Solid Edge part; units mm, degrees
sketch "Sketch1" plane through (0, 0, 0) normal (0, 0, 1) x (1, 0, 0)
  line L0 (-3.8849, 0.05) -> (2.2199, 4.5741)
  line L1 (2.2199, 4.5741) -> (2.2199, -4.4741)
  line L2 (-3.8849, 0.05) -> (2.2199, -4.4741)
extrude "Protrusion1" add sketch "Sketch1" along normal blind 0.1
sketch "Sketch2" plane through (-0.8325, 0.05, 0.1) normal (0, 0, 1) x (0, 1, 0)
  line L0 (-0.79, -3.0024) -> (0.76, -3.0024)
  line L1 (0.76, -3.0024) -> (0.76, -1.0024)
  line L2 (0.76, -1.0024) -> (-0.79, -1.0024)
  line L3 (-0.79, -1.0024) -> (-0.79, -3.0024)
  dimension "D1" = 0.76
  dimension "D2" = 0.79
extrude "Cutout1" cut sketch "Sketch2" against normal through all
Geometry check sheet. Reference: the model listing, model coordinates, mm. Give positions to 0.01 mm unless a question says otherwise; leave off trailing zeros. Order: outer loops, then holes, each group sorted by start corner. A loop starts at its lowest first (then second) coordinate and runs counter-clockwise, first axis right, second up. Notation, with made-up numbers: (12, 77.25) - (19, 77.25) arc R16 cw to (19, 88.25) - close; hole circle Ø7 at (60.25, 50.25). An arc over 180 degrees is marked (long way). Answer as a JSON object with one key per item and string values.
(1) Depth check by flat-ended pin: pin 1 Ø1 at (x, y) = (-2.5, -2) entering from -Z. Enter the tip coordinate at first touch or a pass-through.
Report:
{"pin 1": "through"}
(2) Cross-section at A-A (x = 1.75). Record the cut outline in (y, z).
Report:
{"outline": "(-4.13, 0) - (-0.74, 0) - (-0.74, 0.1) - (-4.13, 0.1) - close; (0.81, 0) - (4.23, 0) - (4.23, 0.1) - (0.81, 0.1) - close"}
(3) Cross-section at B-B (z = 0.05). Record the cut outline in (x, y).
Report:
{"outline": "(-3.88, 0.05) - (2.22, -4.47) - (2.22, 4.57) - close; hole (0.17, -0.74) - (2.17, -0.74) - (2.17, 0.81) - (0.17, 0.81) - close"}
(4) Cross-section at D-D (y = -3.25). Record the cut outline in (x, z).
Report:
{"outline": "(0.57, 0) - (2.22, 0) - (2.22, 0.1) - (0.57, 0.1) - close"}
(5) Cross-section at C-C (x = -3.25). Record the cut outline in (y, z), then the cut area to 3 significant figures.
Report:
{"outline": "(-0.42, 0) - (0.52, 0) - (0.52, 0.1) - (-0.42, 0.1) - close", "area": "0.0941 mm^2"}
(6) Material ranges on line 1 (Y direction, x = 1.5, z = 0.05); line 2 (Y direction, x = -3, z = 0.05); line 3 (X direction, y = -2, z = 0.05), recorded low to high.
Report:
{"line 1": "-3.94 to -0.74, 0.81 to 4.04", "line 2": "-0.61 to 0.71", "line 3": "-1.12 to 2.22"}
